from build123d import *
from OCP.BRepFilletAPI import BRepFilletAPI_MakeChamfer

# Parameters (mm, degrees)
BOSS_EXTRUDE1_DEPTH     = 2.999999969
FILLET1_R               = 6.35
CUT_EXTRUDE1_DEPTH      = 50.956706249
CUT_EXTRUDE1_DEPTH_BACK = 50.956706249
SKETCH2_W               = 12.7
SKETCH2_H               = 38.1
FILLET2_R               = 3.175
CHAMFER1_SIZE           = 3.175
CHAMFER1_SIZE2          = 1.5875
CHAMFER2_SIZE           = 1.5875
CHAMFER2_SIZE2          = 3.175


with BuildPart() as part:
    # Sketch1 → Boss-Extrude1 (new, symmetric)
    with BuildSketch(Plane(origin=(0, 0, 0), x_dir=(0, 0, -1), z_dir=(1, 0, 0))):
        Polygon((-6.35, -25.4), (6.35, -25.4), (6.35, -38.1), (19.05, -38.1), (19.05, -25.4), (19.05, 25.4), (31.75, 25.4), (31.75, 38.1), (-31.75, 38.1), (-31.75, 25.4), (-19.05, 25.4), (-19.05, -25.4), (-19.05, -38.1), (-6.35, -38.1), align=None)
    extrude(amount=BOSS_EXTRUDE1_DEPTH, both=True)

    # Fillet1
    fillet1_edges = [part.edges().sort_by_distance(p)[0] for p in [
        (0, 25.4, -19.05),
        (0, 25.4, 19.05),
        (0, 38.1, 31.75),
        (0, 38.1, -31.75),
    ]]
    fillet(fillet1_edges, radius=FILLET1_R)

    # Sketch2 → Cut-Extrude1 (cut, two sides: drawn at the far end of the back side and taken through both)
    with BuildSketch(Plane(origin=(2.999999969, 0, 0), x_dir=(0, 0, -1), z_dir=(1, 0, 0)).offset(-CUT_EXTRUDE1_DEPTH_BACK)):
        with Locations((0, 6.35)):
            Rectangle(SKETCH2_W, SKETCH2_H)
    extrude(amount=CUT_EXTRUDE1_DEPTH + CUT_EXTRUDE1_DEPTH_BACK, mode=Mode.SUBTRACT)

    # Fillet2
    fillet2_edges = [part.edges().sort_by_distance(p)[0] for p in [
        (0, 25.4, -6.35),
        (0, -12.7, -6.35),
        (0, -12.7, 6.35),
        (0, 25.4, 6.35),
    ]]
    fillet(fillet2_edges, radius=FILLET2_R)

    # Chamfer1: one chamfer whose edges measure the first distance from different faces: ONE call of the kernel's chamfer builder (chamfer() names one face for all edges)
    chamfer1_edges_1 = [part.edges().sort_by_distance(p)[0] for p in [
        (0, -38.1, -6.35),
    ]]
    chamfer1_side_1 = [part.faces().sort_by_distance(p)[0] for p in [
        (0, -31.75, -6.35),
    ]]
    chamfer1_edges_2 = [part.edges().sort_by_distance(p)[0] for p in [
        (0, -38.1, 19.05),
    ]]
    chamfer1_side_2 = [part.faces().sort_by_distance(p)[0] for p in [
        (0, -9.525, 19.05),
    ]]
    chamfer1 = BRepFilletAPI_MakeChamfer(part.part.solid().wrapped)
    for e in chamfer1_edges_1:
        chamfer1.Add(CHAMFER1_SIZE, CHAMFER1_SIZE2, e.wrapped, chamfer1_side_1[0].wrapped)  # the first distance lies on this face
    for e in chamfer1_edges_2:
        chamfer1.Add(CHAMFER1_SIZE, CHAMFER1_SIZE2, e.wrapped, chamfer1_side_2[0].wrapped)  # the first distance lies on this face
    add(Compound.cast(chamfer1.Shape()), mode=Mode.REPLACE)

    # Chamfer2: one chamfer whose edges measure the first distance from different faces: ONE call of the kernel's chamfer builder (chamfer() names one face for all edges)
    chamfer2_edges_1 = [part.edges().sort_by_distance(p)[0] for p in [
        (0, -38.1, -19.05),
    ]]
    chamfer2_side_1 = [part.faces().sort_by_distance(p)[0] for p in [
        (0, -38.1, -13.49375),
    ]]
    chamfer2_edges_2 = [part.edges().sort_by_distance(p)[0] for p in [
        (0, -38.1, 6.35),
    ]]
    chamfer2_side_2 = [part.faces().sort_by_distance(p)[0] for p in [
        (0, -38.1, 11.90625),
    ]]
    chamfer2 = BRepFilletAPI_MakeChamfer(part.part.solid().wrapped)
    for e in chamfer2_edges_1:
        chamfer2.Add(CHAMFER2_SIZE, CHAMFER2_SIZE2, e.wrapped, chamfer2_side_1[0].wrapped)  # the first distance lies on this face
    for e in chamfer2_edges_2:
        chamfer2.Add(CHAMFER2_SIZE, CHAMFER2_SIZE2, e.wrapped, chamfer2_side_2[0].wrapped)  # the first distance lies on this face
    add(Compound.cast(chamfer2.Shape()), mode=Mode.REPLACE)


solid = part.part
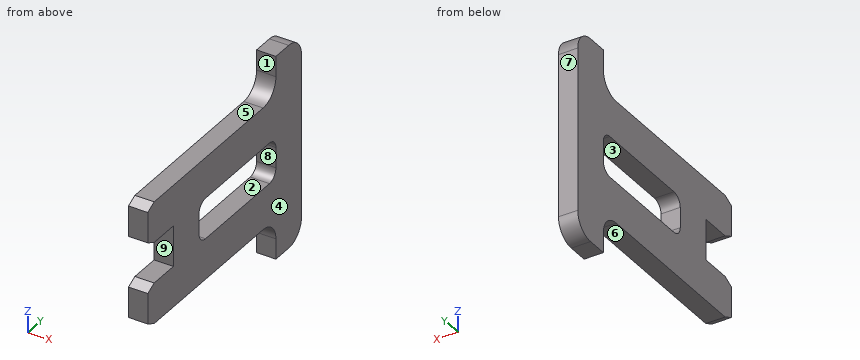
Design review of the part built by this model. Coordinates are the model's own, in mm. Face numbers are marked on the shaded views. A direction names the side the tool comes from. Give positions to 0.01 mm unless a question says otherwise; leave off trailing zeros. Order: outer loops, then holes, each group sorted by start corner. A loop starts at its lowest first (then second) coordinate and runs counter-clockwise, first axis right, second up.
1. To check wall thickness, follow L1, parallel to Z at x = 0.85, y = -29; L2, parallel to Y at x = -2.15, z = 2. State the ranges of each line that lie inside material, in increasing order.
Solution:
L1: z = -19.05 to -6.35, 6.35 to 19.05
L2: y = -25.4 to -12.7, 25.4 to 38.1
2. Add section A-A, the plane y = -31.5. State the section outline as (x, z) points.
Solution:
outline: (-3, -19.05) - (3, -19.05) - (3, -6.35) - (-3, -6.35) - close; (-3, 6.35) - (3, 6.35) - (3, 19.05) - (-3, 19.05) - close
3. Add section C-C, the plane y = 21. State the section outline as (x, z) points.
Solution:
outline: (-3, -19.36) - (3, -19.36) - (3, -6.35) - (-3, -6.35) - close; (-3, 6.35) - (3, 6.35) - (3, 19.36) - (-3, 19.36) - close
4. Tool access review of the marked faces 5, 6, 7, 8 and 9: name each direction out of +Z, -Z, +X, -X, +Y, -Y from which nothing blocks a thin tool from reaching the whole face with its end or side.
Solution:
face 5: +Z, +X, -X, -Y
face 6: -Z, +X, -X, -Y
face 7: +Z, -Z, +X, -X, +Y
face 8: +X, -X
face 9: +X, -X, -Y
5. Mouldability with a two-part tool opening along Y and no side actions: class the marked faces 1, 2, 3 and 4 as +Y half, -Y half, draft (parallel to the pull), parting line (faces both ways), or undercut.
Solution:
face 1: -Y half
face 2: undercut
face 3: undercut
face 4: draft
6. Add section D-D, the plane y = -15. State the section outline as (x, z) points, then the cut area to 3 significant figures.
Solution:
outline: (-3, -19.05) - (3, -19.05) - (3, 19.05) - (-3, 19.05) - close
area: 229 mm2
7. For pin 1 Ø1.8 at (x, y) = (0.5, -12) entering from +Z; pin 2 Ø3 at (x, y) = (0.5, -21) entering from -Z; pin 3 Ø1.8 at (x, z) = (1.5, 29) entering from -Y, all flat-tipped, find the tip position at first contact; note any pin that passes through.
Solution:
pin 1: stops at z = 19.05
pin 2: stops at z = -19.05
pin 3: stops at y = 25.4
